```python
from build123d import *

# Parameters (mm, degrees)
CROQUIS1_R              = 1.58
CROQUIS1_R_2            = 14.25
SALIENTE_EXTRUIR1_DEPTH = 4


with BuildPart() as part:
    # Croquis1 → Saliente-Extruir1 (new body)
    with BuildSketch(Plane.XY):
        with BuildLine():
            Line((30.124466094, -7.785533906), (37.91, 0))
            Line((37.91, 0), (97.165453192, 63.015199165))
            ThreePointArc((97.165453192, 63.015199165), (101.36659613, 64.558696549), (105.120132173, 62.12087922))
            Line((105.120132173, 62.12087922), (141.58, 0))
            Line((141.58, 0), (153.799494633, -22.164589344))
            Line((153.799494633, -22.164589344), (155.71, -25.63))
            Line((155.71, -25.63), (163.352260057, -39.49207539))
            ThreePointArc((163.352260057, -39.49207539), (187.721004887, -48.471027794), (200.08, -25.63))
            Line((200.08, -25.63), (113.076169939, 130.225021029))
            ThreePointArc((113.076169939, 130.225021029), (109.214360618, 132.762403753), (104.922096847, 131.051160333))
            Line((104.922096847, 131.051160333), (0, 9.25))
            Line((0, 9.25), (-35, 9.25))
            Line((-35, 9.25), (-50, 9.25))
            Line((-50, 9.25), (-50, -9.25))
            Line((-50, -9.25), (-35, -9.25))
            Line((-35, -9.25), (0, -9.25))
            Line((0, -9.25), (26.588932188, -9.25))
            ThreePointArc((26.588932188, -9.25), (28.50234935, -8.869397663), (30.124466094, -7.785533906))
        make_face()
        with Locations((-35, 0)):
            Circle(CROQUIS1_R, mode=Mode.SUBTRACT)
        Circle(CROQUIS1_R, mode=Mode.SUBTRACT)
        with Locations((178.55, -25.63)):
            Circle(CROQUIS1_R_2, mode=Mode.SUBTRACT)
    extrude(amount=SALIENTE_EXTRUIR1_DEPTH)


solid = part.part
```
Read the model definition and answer for the solid it produces. Units are mm, in the model's axes. A direction names the side the tool comes from. Give positions to 0.01 mm unless a question says otherwise; leave off trailing zeros. Order: outer loops, then holes, each group sorted by start corner. A loop starts at its lowest first (then second) coordinate and runs counter-clockwise, first axis right, second up.
(1) Straight lines are drawn through the part: L1, parallel to Y at x = -35, z = 1.8; L2, parallel to X at y = -19, z = 2. For each, find the intervals that lie inside material, in ascending order.
(2) Find section A-A (z = 1.85). Give the vertices of the cut face in (x, y), plus the area to 3 significant figures.
(3) For faces 5 (the flat face through (84, 55, 0)), 6 (the flat face through (33.96, -3.95, 1.97)), determine the directions among +Z, -Z, +X, -X, +Y, -Y from which every point of the face is accessible in a straight line to the end or side of a thin tool.
(4) For a pull along Y with two mould halves and no side action, classify faces 1 (the flat face through (67.123, 31.066, 1.972)), 2 (the flat face through (84, 55, 4)), 3 (the cylindrical face through (167.24, -34.3, 1.97)), 4 (the flat face through (53.196, 71.003, 1.972)) as released by +Y, released by -Y, zero draft, split by the parting line, or undercut.
(5) Given pin 1 (1 mm diameter, centred on y = 73, z = 1, fed in from +X), flat-ended and moving along its own axis, determine where the tip first touches the part or whether it passes through.
(6) Find section B-B (y = 57). Give the vertices of the cut face in (x, z), plus the area to 3 significant figures.
(7) Find section D-D (x = 82.5). Give the vertices of the cut face in (y, z).
(8) Find section C-C (x = 178.55). Give the vertices of the cut face in (y, z), plus the area to 3 significant figures.
Result sheet:
1. L1: y = -9.25 to -1.58, 1.58 to 9.25
1. L2: x = 152.05 to 165.94, 191.16 to 196.38
2. outline: (-50, -9.25) - (26.59, -9.25) arc R5 ccw to (30.12, -7.79) - (37.91, 0) - (97.17, 63.02) arc R5 cw to (105.12, 62.12) - (141.58, 0) - (163.35, -39.49) arc R19.83 ccw to (200.08, -25.63) - (113.08, 130.23) arc R5 ccw to (104.92, 131.05) - (0, 9.25) - (-50, 9.25) - close; hole circle Ø3.16 at (-35, 0); hole circle Ø3.16 at (0, 0); hole circle Ø28.5 at (178.55, -25.63)
2. area: 12,200 mm2
3. face 5: -Z, +X, -X, +Y, -Y
3. face 6: +Z, -Z, -Y
4. face 1: released by -Y
4. face 2: zero draft
4. face 3: undercut
4. face 4: released by +Y
5. pin 1: stops at x = 145.3
6. outline: (41.13, 0) - (91.51, 0) - (91.51, 4) - (41.13, 4) - close; (108.13, 0) - (153.95, 0) - (153.95, 4) - (108.13, 4) - close
6. area: 385 mm2
7. outline: (47.42, 0) - (105.02, 0) - (105.02, 4) - (47.42, 4) - close
8. outline: (-49.63, 0) - (-39.88, 0) - (-39.88, 4) - (-49.63, 4) - close; (-11.38, 0) - (12.94, 0) - (12.94, 4) - (-11.38, 4) - close
8. area: 136 mm2
